```python
from build123d import *

# Parameters (mm, degrees)
SKETCH1_W           = 25.4
SKETCH1_H           = 3.175
BOSS_EXTRUDE1_DEPTH = 1.5875


with BuildPart() as part:
    # Sketch1 → Boss-Extrude1 (new body, symmetric)
    with BuildSketch(Plane(origin=(0, 0, 0), x_dir=(1, 0, 0), z_dir=(0, 1, 0))):
        Polygon((-101.6, -12.7), (-101.6, -88.9), (-63.5, -88.9), (-38.1, -88.9), (-12.7, -88.9), (12.7, -88.9), (38.1, -88.9), (63.5, -88.9), (101.6, -88.9), (101.6, -12.7), (104.775, -12.7), (104.775, -38.1), (107.95, -38.1), (107.95, 88.9), (-107.95, 88.9), (-107.95, -38.1), (-104.775, -38.1), (-104.775, -12.7), align=None)
        with Locations((-50.8, -90.4875)):
            Rectangle(SKETCH1_W, SKETCH1_H)
        with Locations((0, -90.4875)):
            Rectangle(SKETCH1_W, SKETCH1_H)
        with Locations((50.8, -90.4875)):
            Rectangle(SKETCH1_W, SKETCH1_H)
    extrude(amount=BOSS_EXTRUDE1_DEPTH, both=True)


solid = part.part
```
Work out the finished part from the listing and answer in its coordinate system (mm). Coordinates: 2 decimals unless noted, no trailing zeros. Write each loop counter-clockwise with the first axis right and the second up, starting at its lowest first coordinate (ties: lowest second). Pieces come first, ordered by that corner, then holes. Notation, with made-up numbers: (68.25, -3) - (77.25, -3) arc R21 ccw to (77.25, 23) - close; hole circle Ø3 at (88.5, -2). An arc over 180 degrees is marked (long way). Answer as a JSON object with one key per item and string values.
Q1. Find section C-C (x = -70). Write down the section's boundary in (y, z), plus the area to 3 significant figures.
Results list:
{"outline": "(-1.59, -88.9) - (1.59, -88.9) - (1.59, 88.9) - (-1.59, 88.9) - close", "area": "565 mm^2"}
Q2. Find section A-A (z = 16.5). State how many separate pieces and enclosed holes the cut face has, plus the area to 3 significant figures.
Results list:
{"separate pieces": "3", "enclosed holes": "0", "area": "665 mm^2"}
Q3. Consider L1, parallel to X at y = -0.4, z = 17 (3 decimals); L2, parallel to Z at x = 20, y = -1.4; L3, parallel to X at y = 0.8, z = 49.5. Determine where each line is inside the solid, lowest interval first. Write a range as from..to.
Results list:
{"L1": "x = -107.95..-104.775, -101.6..101.6, 104.775..107.95", "L2": "z = -88.9..88.9", "L3": "x = -101.6..101.6"}
Q4. Find section B-B (y = -1.1). Write down the section's boundary in (x, z) (3 decimals).
Results list:
{"outline": "(-107.95, -88.9) - (107.95, -88.9) - (107.95, 38.1) - (104.775, 38.1) - (104.775, 12.7) - (101.6, 12.7) - (101.6, 88.9) - (63.5, 88.9) - (63.5, 92.075) - (38.1, 92.075) - (38.1, 88.9) - (12.7, 88.9) - (12.7, 92.075) - (-12.7, 92.075) - (-12.7, 88.9) - (-38.1, 88.9) - (-38.1, 92.075) - (-63.5, 92.075) - (-63.5, 88.9) - (-101.6, 88.9) - (-101.6, 12.7) - (-104.775, 12.7) - (-104.775, 38.1) - (-107.95, 38.1) - close"}
Q5. Find section D-D (z = 45.5). Write down the section's boundary in (x, y).
Results list:
{"outline": "(-101.6, -1.59) - (101.6, -1.59) - (101.6, 1.59) - (-101.6, 1.59) - close"}
Q6. Given pin 1 Ø1.6 at (y, z) = (-0.5, 91) entering from +X; pin 2 Ø1.5 at (x, y) = (-28, 1) entering from +Z; pin 3 Ø1 at (y, z) = (-1, 90) entering from -X, each flat-ended and moving along its own axis, determine where each tip first touches the part or whether it passes through.
Results list:
{"pin 1": "stops at x = 63.5", "pin 2": "stops at z = 88.9", "pin 3": "stops at x = -63.5"}
